```python
from build123d import *

# Parameters (mm, degrees)
SKETCH1_W                 = 24
SKETCH1_H                 = 135
BOSS_EXTRUDE1_DEPTH       = 10
M5X0_8_TAPPED_HOLE1_D     = 4.2
M5X0_8_TAPPED_HOLE1_DEPTH = 12.4
M5X0_8_TAPPED_HOLE1_TIP   = 1.2618073
M5X0_8_TAPPED_HOLE2_D     = 4.2
M5X0_8_TAPPED_HOLE2_DEPTH = 12.4
M5X0_8_TAPPED_HOLE2_TIP   = 1.2618073
M3X0_5_TAPPED_HOLE1_D     = 2.5


with BuildPart() as part:
    # Sketch1 → Boss-Extrude1 (new body)
    with BuildSketch(Plane(origin=(0, 0, 0), x_dir=(1, 0, 0), z_dir=(0, 1, 0))):
        with Locations((12, 0)):
            Rectangle(SKETCH1_W, SKETCH1_H)
    extrude(amount=BOSS_EXTRUDE1_DEPTH)

    # M5x0.8 Tapped Hole1
    with Locations(Plane(origin=(24, 0, 0), x_dir=(0, 0, -1), z_dir=(1, 0, 0))):
        with Locations((0, 5), (-50, 5), (50, 5)):
            Hole(M5X0_8_TAPPED_HOLE1_D / 2, depth=M5X0_8_TAPPED_HOLE1_DEPTH)
            with Locations((0, 0, -(M5X0_8_TAPPED_HOLE1_DEPTH + M5X0_8_TAPPED_HOLE1_TIP / 2))):  # 118° drill point
                Cone(0, M5X0_8_TAPPED_HOLE1_D / 2, M5X0_8_TAPPED_HOLE1_TIP, mode=Mode.SUBTRACT)

    # M5x0.8 Tapped Hole2
    with Locations(Plane.ZY):
        with Locations((50, 5), (0, 5), (-50, 5)):
            Hole(M5X0_8_TAPPED_HOLE2_D / 2, depth=M5X0_8_TAPPED_HOLE2_DEPTH)
            with Locations((0, 0, -(M5X0_8_TAPPED_HOLE2_DEPTH + M5X0_8_TAPPED_HOLE2_TIP / 2))):  # 118° drill point
                Cone(0, M5X0_8_TAPPED_HOLE2_D / 2, M5X0_8_TAPPED_HOLE2_TIP, mode=Mode.SUBTRACT)

    # M3x0.5 Tapped Hole1 (through all)
    with Locations(Plane(origin=(0, 10, 0), x_dir=(-1, 0, 0), z_dir=(0, 1, 0))):
        with Locations((-5, -7.5), (-5, 7.5)):
            Hole(M3X0_5_TAPPED_HOLE1_D / 2)


solid = part.part
```
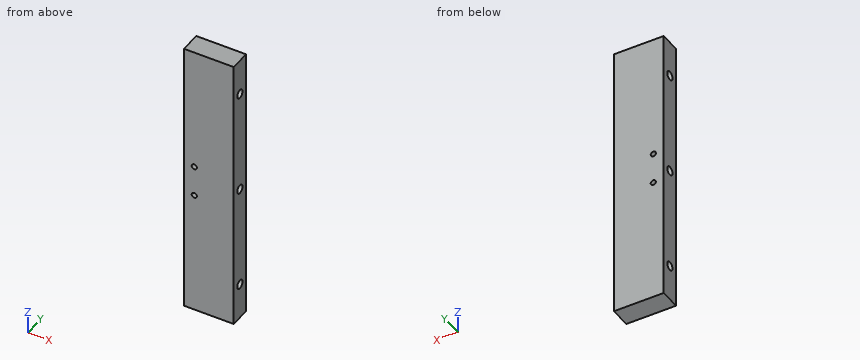
Design review of the part built by this model. Coordinates are the model's own, in mm. Round coordinates to 2 decimals unless told otherwise and drop trailing zeros. Order: outer loops, then holes, each group sorted by start corner. A loop starts at its lowest first (then second) coordinate and runs counter-clockwise, first axis right, second up. Notation, with made-up numbers: (44, 70) - (67, 70) arc R15 cw to (67, 80) - close; hole circle Ø6 at (-11, 58). An arc over 180 degrees is marked (long way). Return JSON: item names as keys, results as strings.
Q1. Consider section B-B on z = 0. Write out the cut boundary in (x, y), plus the area to 3 significant figures.
Computed values:
{"outline": "(0, 0) - (24, 0) - (24, 2.9) - (0, 2.9) - close; (0, 7.1) - (24, 7.1) - (24, 10) - (0, 10) - close", "area": "139 mm2"}
Q2. For pin 1 Ø4 at (y, z) = (5, 0) entering from +X, flat-tipped, find the tip position at first contact; note if it passes through.
Computed values:
{"pin 1": "passes through"}
Q3. Wall thickness on L1, parallel to Z at x = 19, y = 5; L2, parallel to Y at x = 6.5, z = -50; L3, parallel to Z at x = 3, y = 6.25: over which ranges is each line inside the solid? List them lowest first. Write a range as [from, to].
Computed values:
{"L1": "z = [-67.5, -52.1], [-47.9, -2.1], [2.1, 47.9], [52.1, 67.5]", "L2": "y = [0, 2.9], [7.1, 10]", "L3": "z = [-67.5, -51.69], [-48.31, -1.69], [1.69, 48.31], [51.69, 67.5]"}
Q4. Consider section A-A on x = 5. Write out the cut boundary in (y, z).
Computed values:
{"outline": "(0, -67.5) - (10, -67.5) - (10, -8.75) - (0, -8.75) - close; (0, -6.25) - (10, -6.25) - (10, 6.25) - (0, 6.25) - close; (0, 8.75) - (10, 8.75) - (10, 67.5) - (0, 67.5) - close; hole circle Ø4.2 at (5, -50); hole circle Ø4.2 at (5, 0); hole circle Ø4.2 at (5, 50)"}
Q5. Consider section C-C on x = 14. Write out the cut boundary in (y, z), plus the area to 3 significant figures.
Computed values:
{"outline": "(0, -67.5) - (10, -67.5) - (10, 67.5) - (0, 67.5) - close; hole circle Ø4.2 at (5, -50); hole circle Ø4.2 at (5, 0); hole circle Ø4.2 at (5, 50)", "area": "1,310 mm2"}
